from build123d import *

# Parameters (mm, degrees)
EXTRUDE_1_DEPTH = 1
EXTRUDE_2_DEPTH = 1


with BuildPart() as part:
    # 草图1 → 凸台-拉伸1 (new body)
    with BuildSketch(Plane(origin=(0, 0, 0), x_dir=(1, 0, 0), z_dir=(0, 1, 0))):
        Polygon((2.736696129, 9.473412041), (16.58017542, 72.883143872), (77.860885248, -1.274015551), (79.4026, -1.274015551), (79.4026, -4.17), (1.5, -4.17), (1.5, 3.808754461), align=None)
    extrude(amount=EXTRUDE_1_DEPTH)

    # 草图2 → 凸台-拉伸2 (add)
    # profile 1 of 2: a face of its own
    with BuildSketch(Plane.XZ.offset(-1)):
        with BuildLine():
            Line((27.247178656, -37.134108742), (26.498069264, -37.184070121))
            Line((26.498069264, -37.184070121), (26.367735231, -35.229871707))
            add(Edge.make_bspline(
                [(26.367735231, -35.229871707), (26.336136972, -35.237959723), (26.270940383, -35.254647701), (26.168685096, -35.271305323), (26.06001111, -35.283910157), (25.985459776, -35.288939032), (25.947055355, -35.291529611)],
                knots=[0, 0, 0, 0, 0.918524269, 1.895188248, 2.915725933, 4, 4, 4, 4], degree=3))
            add(Edge.make_bspline(
                [(25.947055355, -35.291529611), (25.888971534, -35.295059263), (25.773910138, -35.302051343), (25.602623819, -35.297682043), (25.435001026, -35.282463383), (25.271332319, -35.25320731), (25.111285307, -35.21277006), (24.954612218, -35.160015392), (24.802048503, -35.094230317), (24.653616239, -35.017919209), (24.513272279, -34.927178562), (24.389160738, -34.815143767), (24.279568532, -34.686737032), (24.186443183, -34.540279182), (24.109248199, -34.376664865), (24.048793797, -34.195673673), (24.00163799, -33.997727925), (23.98455536, -33.858833633), (23.975706741, -33.786887875)],
                knots=[0, 0, 0, 0, 0.996278886, 1.973582945, 2.931399707, 3.876509745, 4.818088033, 5.756508938, 6.704738743, 7.661035354, 8.613001496, 9.557911395, 10.514025425, 11.496214958, 12.521468463, 13.604750262, 14.759286266, 16, 16, 16, 16], degree=3))
            add(Edge.make_bspline(
                [(23.975706741, -33.786887875), (23.973452918, -33.730795501), (23.969040147, -33.620971923), (23.981295878, -33.459643046), (24.008316205, -33.30606268), (24.051249008, -33.160965902), (24.106879389, -33.024846473), (24.176026658, -32.899197677), (24.256208333, -32.783062463), (24.320948784, -32.715703234), (24.35321277, -32.682134156)],
                knots=[0, 0, 0, 0, 1.117887841, 2.188718949, 3.216803733, 4.219776148, 5.198259829, 6.140927987, 7.073514742, 8, 8, 8, 8], degree=3))
            add(Edge.make_bspline(
                [(24.35321277, -32.682134156), (24.390372306, -32.647075002), (24.465903781, -32.575812818), (24.597971222, -32.486883084), (24.743773905, -32.407877723), (24.905322916, -32.340638498), (25.082570482, -32.286184948), (25.274941514, -32.242813813), (25.482676378, -32.20986596), (25.626939116, -32.198747031), (25.701450626, -32.193004119)],
                knots=[0, 0, 0, 0, 0.835515405, 1.698291186, 2.597844701, 3.548800166, 4.558778601, 5.631012435, 6.776421119, 8, 8, 8, 8], degree=3))
            add(Edge.make_bspline(
                [(25.701450626, -32.193004119), (25.763647746, -32.18990621), (25.884969005, -32.183863452), (26.061872954, -32.178079125), (26.228994693, -32.176297304), (26.386085383, -32.175276922), (26.533358419, -32.180136733), (26.671037915, -32.185786151), (26.798547568, -32.19637649), (26.880137368, -32.205823077), (26.919139372, -32.210338786)],
                knots=[0, 0, 0, 0, 1.225714187, 2.39086934, 3.483452773, 4.515316552, 5.482438301, 6.383408239, 7.227227922, 8, 8, 8, 8], degree=3))
            Line((26.919139372, -32.210338786), (27.247178656, -37.134108742))
        make_face()
        with BuildLine():
            add(Edge.make_bspline(
                [(26.205686584, -32.800151678), (26.176079833, -32.796164938), (26.108374661, -32.787048001), (25.99329716, -32.783062649), (25.852753393, -32.782701532), (25.750681695, -32.786552967), (25.695306953, -32.788642403)],
                knots=[0, 0, 0, 0, 0.700870625, 1.60276173, 2.699478359, 4, 4, 4, 4], degree=3))
            add(Edge.make_bspline(
                [(25.695306953, -32.788642403), (25.657932433, -32.791833077), (25.58475194, -32.798080519), (25.478477782, -32.816141959), (25.378387391, -32.84124998), (25.283896528, -32.871209194), (25.196224059, -32.909838569), (25.115210741, -32.955481345), (25.03925353, -33.006155967), (24.970876759, -33.065156289), (24.909669441, -33.130586372), (24.856775337, -33.202660022), (24.814150815, -33.281632292), (24.778453834, -33.366335047), (24.754586229, -33.458484944), (24.738023638, -33.556671393), (24.729630946, -33.661109096), (24.731926616, -33.732692134), (24.733106875, -33.769494709)],
                knots=[0, 0, 0, 0, 1.15558629, 2.262674533, 3.317300313, 4.333814689, 5.313668358, 6.26345259, 7.196628822, 8.12266155, 9.039750842, 9.952722527, 10.868938376, 11.799486507, 12.778234057, 13.794331363, 14.866012282, 16, 16, 16, 16], degree=3))
            add(Edge.make_bspline(
                [(24.733106875, -33.769494709), (24.737096219, -33.808354477), (24.744855943, -33.883941104), (24.765532333, -33.993323197), (24.796982251, -34.094527148), (24.834175778, -34.189173984), (24.883030807, -34.274790461), (24.938222836, -34.354330579), (25.003166703, -34.425471317), (25.076160949, -34.48869148), (25.15623493, -34.544138738), (25.243910401, -34.590592199), (25.33838039, -34.628357489), (25.438808525, -34.659340274), (25.546631026, -34.679604309), (25.6607371, -34.69332827), (25.781865267, -34.696662397), (25.864468434, -34.693317664), (25.906870167, -34.69160075)],
                knots=[0, 0, 0, 0, 1.106707454, 2.152670698, 3.147355285, 4.106207412, 5.027575719, 5.933648193, 6.84458558, 7.748722376, 8.664759674, 9.598405993, 10.553638462, 11.544030495, 12.57124846, 13.657767573, 14.797688756, 16, 16, 16, 16], degree=3))
            add(Edge.make_bspline(
                [(25.906870167, -34.69160075), (25.948454683, -34.689062607), (26.027460929, -34.684240401), (26.139157586, -34.670071787), (26.238651685, -34.652463648), (26.299233543, -34.633690353), (26.327848462, -34.624823072)],
                knots=[0, 0, 0, 0, 1.169113496, 2.221193815, 3.159807954, 4, 4, 4, 4], degree=3))
            Line((26.327848462, -34.624823072), (26.205686584, -32.800151678))
        make_face(mode=Mode.SUBTRACT)
    # profile 2 of 2: a face of its own
    with BuildSketch(Plane.XZ.offset(-1)):
        with BuildLine():
            Line((27.935432574, -32.083430945), (28.691055961, -32.033035119))
            Line((28.691055961, -32.033035119), (28.892204819, -35.049014672))
            add(Edge.make_bspline(
                [(28.892204819, -35.049014672), (28.897507047, -35.108369157), (28.90777105, -35.223266999), (28.932979911, -35.388569892), (28.964110993, -35.541441954), (29.003735435, -35.681075959), (29.049877232, -35.80835476), (29.1038274, -35.922731741), (29.166322232, -36.023827925), (29.235308242, -36.112819124), (29.311927252, -36.188595136), (29.393405004, -36.254014097), (29.481306787, -36.307626326), (29.575139181, -36.34943819), (29.674153705, -36.380669278), (29.77898, -36.398543183), (29.88926244, -36.40743298), (29.964575532, -36.403749393), (30.003206868, -36.401859922)],
                knots=[0, 0, 0, 0, 1.439721744, 2.786999531, 4.038482243, 5.207354554, 6.291223817, 7.306895795, 8.257373748, 9.158006139, 10.021101694, 10.855396504, 11.677909811, 12.501584238, 13.332400486, 14.17961271, 15.066244781, 16, 16, 16, 16], degree=3))
            add(Edge.make_bspline(
                [(30.003206868, -36.401859922), (30.038729559, -36.398923305), (30.108621995, -36.393145384), (30.209684602, -36.370152125), (30.305513155, -36.33941236), (30.39396647, -36.294571366), (30.477851847, -36.242257996), (30.554413819, -36.177580795), (30.625625293, -36.103498895), (30.690312721, -36.018648553), (30.748019791, -35.922099382), (30.795846408, -35.813332953), (30.835215343, -35.692799841), (30.864869703, -35.56043382), (30.885460677, -35.416124074), (30.896184878, -35.260061022), (30.900103493, -35.091966457), (30.894877985, -34.976148439), (30.89216671, -34.916055829)],
                knots=[0, 0, 0, 0, 0.874153846, 1.719935635, 2.538919661, 3.33858121, 4.148201754, 4.961360028, 5.792268906, 6.667174948, 7.575383943, 8.547579609, 9.578266644, 10.684296341, 11.873995655, 13.154059738, 14.523373295, 16, 16, 16, 16], degree=3))
            Line((30.89216671, -34.916055829), (30.690852339, -31.899659959))
            Line((30.690852339, -31.899659959), (31.446475726, -31.849264133))
            Line((31.446475726, -31.849264133), (31.644583456, -34.819645723))
            add(Edge.make_bspline(
                [(31.644583456, -34.819645723), (31.648578386, -34.909049834), (31.656279514, -35.081396411), (31.647945267, -35.331247935), (31.626567199, -35.562863946), (31.588387672, -35.776491181), (31.535946157, -35.972611101), (31.467518593, -36.150749447), (31.382473647, -36.310338583), (31.282123362, -36.451459106), (31.168931277, -36.575879794), (31.045026327, -36.685519975), (30.909366494, -36.779545606), (30.762799952, -36.858191677), (30.605635955, -36.922509938), (30.437166438, -36.970123465), (30.258184476, -37.004084934), (30.134610832, -37.01396111), (30.071432155, -37.019010437)],
                knots=[0, 0, 0, 0, 1.392410449, 2.68418501, 3.887439475, 5.009764914, 6.057622654, 7.042685123, 7.97321012, 8.864539029, 9.730657168, 10.585789343, 11.434193697, 12.293614102, 13.169840523, 14.071727903, 15.014145116, 16, 16, 16, 16], degree=3))
            add(Edge.make_bspline(
                [(30.071432155, -37.019010437), (30.005641486, -37.022210067), (29.876827974, -37.028474717), (29.687187359, -37.019546443), (29.506284369, -36.993457544), (29.334867231, -36.949141616), (29.172110457, -36.889501605), (29.017921074, -36.813602283), (28.873390267, -36.719534025), (28.737918252, -36.609392285), (28.612277586, -36.481652914), (28.503727367, -36.331489281), (28.405978482, -36.163774568), (28.323255189, -35.975917378), (28.255263986, -35.767835389), (28.199330237, -35.541157099), (28.158249949, -35.294314561), (28.141696756, -35.123047155), (28.133118143, -35.034288632)],
                knots=[0, 0, 0, 0, 1.000276318, 1.958470843, 2.879248422, 3.77219387, 4.643297829, 5.508534547, 6.377296365, 7.25736848, 8.156904209, 9.090557831, 10.064428775, 11.101560789, 12.202301066, 13.386404782, 14.645516639, 16, 16, 16, 16], degree=3))
            Line((28.133118143, -35.034288632), (27.935432574, -32.083430945))
        make_face()
    extrude(amount=-EXTRUDE_2_DEPTH)


solid = part.part
Geometry: final body of the model. Coordinates: model frame, mm. Coordinates: 2 decimals unless noted, no trailing zeros. Order: outer loops, then holes, each group sorted by start corner. A loop starts at its lowest first (then second) coordinate and runs counter-clockwise, first axis right, second up.
(1) Section query A-A (y = 1.65). State how many separate pieces and enclosed holes the cut face has, plus the area to 3 significant figures.
(2) Section query B-B (x = 47). Return the cut outline in (y, z), plus the area to 3 significant figures.
(3) Section query C-C (z = -49.5). Return the cut outline in (x, y), plus the area to 3 significant figures.
(4) Material intervals for probe 1 along X at (y, z) = (1.1, -33); probe 2 along Y at (x, z) = (37, -44); probe 3 along Z at (x, y) = (66, 0.45), sorted ascending.
(5) First-contact query: pin 1 (0.8 mm diameter, centred on x = 25.5, z = -33.5, fed in from +Y); pin 2 (0.8 mm diameter, centred on x = 78.5, y = 0.5, fed in from -Z). Flat tips, straight axial feed; report the tip coordinate or a pass-through.
Solution:
1. separate pieces: 2
1. enclosed holes: 1
1. area: 15.4 mm2
2. outline: (0, -36.07) - (1, -36.07) - (1, 4.17) - (0, 4.17) - close
2. area: 40.2 mm2
3. outline: (11.48, 0) - (35.9, 0) - (35.9, 1) - (11.48, 1) - close
3. area: 24.4 mm2
4. probe 1: x = 24.12 to 25.05, 26.22 to 26.97, 28 to 28.76, 30.76 to 31.52
4. probe 2: y = 0 to 1
4. probe 3: z = -13.08 to 4.17
5. pin 1: stops at y = 1
5. pin 2: stops at z = 1.27
